Autodesk Fusion 360 part; units mm, degrees
sketch "Sketch1" plane through (0, 0, 0) normal (0, 0, 1) x (1, 0, 0)
  line L0 (0, 0) -> (51.8, 0)
  line L1 (51.8, 0) -> (51.8, 24.3)
  line L2 (51.8, 24.3) -> (0, 24.3)
  line L3 (0, 24.3) -> (0, 0)
  circle A0 centre (14, 5.4) radius 1.6
  circle A1 centre (38.7, 17.8) radius 1.6
  circle A2 centre (38.7, 5.4) radius 1.6
  line L4 (38.7, 17.8) -> (38.7, 5.4) construction
  line L5 (38.7, 5.4) -> (14, 5.4) construction
  line L6 (25.9, 24.3) -> (25.9, 0) construction
  circle A3 centre (38.7, 17.8) radius 3
  circle A4 centre (38.7, 5.4) radius 3
  circle A5 centre (14, 5.4) radius 3
  line L7 (51.8, 0) -> (59, 4.65)
  line L8 (59, 4.65) -> (59, 19.65)
  line L9 (59, 19.65) -> (51.8, 24.3)
  line L10 (0, 0) -> (-7.2, 4.65)
  line L11 (-7.2, 4.65) -> (-7.2, 19.65)
  line L12 (-7.2, 19.65) -> (0, 24.3)
  circle A6 centre (54.8, 12.15) radius 1.6
  circle A7 centre (-3, 12.15) radius 1.6
  line L13 (0, 12.15) -> (51.8, 12.15) construction
  circle A8 centre (-3, 12.15) radius 3
  circle A9 centre (54.8, 12.15) radius 3
  line L14 (-7.2, 4.65) -> (-10.8, 6.975)
  line L15 (-10.8, 6.975) -> (-10.8, 17.325)
  line L16 (-10.8, 17.325) -> (-8, 19.1333)
  line L17 (-8, 19.1333) -> (-8, 17.1333)
  line L18 (-8, 17.1333) -> (-8.8, 17.1333)
  line L19 (-8.8, 17.1333) -> (-8.8, 8.0642)
  line L20 (-8.8, 8.0642) -> (-7.2, 7.0308)
  dimension "d1" = 3.2
  dimension "d2" = 24.7
  dimension "d3" = 12.4
  dimension "d4" = 51.8
  dimension "d5" = 24.3
  dimension "d6" = 11.9
  dimension "d7" = 5.4
  dimension "d8" = 6
  dimension "d13" = 3.2
  dimension "d14" = 1.2
  dimension "d15" = 1.2
  dimension "d16" = 15
  dimension "d35" = 2
  dimension "d36" = 2
  dimension "d37" = 1.6
  dimension "d38" = 0.8
  dimension "d39" = 2
extrude "Extrude1" add sketch "Sketch1" along normal blind 5.6 contours L0 L1 L2 L3 | L3 L10 L11 L12 | L1 L7 L8 L9 | L11 L14 L15 L16 L17 L18 L19 L20
extrude "Extrude2" add sketch "Sketch1" along normal blind 2.5 contours A3 | A4 | A5
extrude "Extrude3" add sketch "Sketch1" along normal blind 2.6 from surface at 3 contours A8 | A9
sketch "Sketch2" plane through (0, 0, 5.6) normal (0, 0, 1) x (-1, 0, 0)
  circle A0 centre (-14, -5.4) radius 3
  circle A1 centre (-38.7, -17.8) radius 3
  circle A2 centre (-38.7, -5.4) radius 3
  line L0 (0, 0) -> (-51.8, 0)
  line L1 (-51.8, -24.3) -> (0, -24.3)
  line L2 (0, -24.3) -> (7.2, -19.65)
  line L3 (7.2, -19.65) -> (7.2, -7.0308)
  line L4 (10.8, -6.975) -> (0, 0)
  line L5 (-59.2, -13.3404) -> (7.2, -13.3404) construction
  line L6 (-59.2, -17.3404) -> (7.2, -17.3404)
  line L7 (7.2, -9.3404) -> (-59.2, -9.3404)
  line L8 (-51.5, -9.3404) -> (-51.5, -17.3404)
  line L9 (-0.5, -9.3404) -> (-0.5, -17.3404)
  line L10 (7.2, -7.0308) -> (8.8, -8.0642)
  line L11 (8.8, -8.0642) -> (8.8, -17.1333)
  line L12 (8.8, -17.1333) -> (8, -17.1333)
  line L13 (8, -17.1333) -> (8, -19.1333)
  line L14 (8, -19.1333) -> (10.8, -17.325)
  line L15 (10.8, -17.325) -> (10.8, -6.975)
  line L16 (-51.8, 0) -> (-59, -4.65)
  line L17 (-59, -4.65) -> (-59, -19.65)
  line L18 (-59, -19.65) -> (-51.8, -24.3)
  circle A3 centre (-54.8, -12.15) radius 1.6
  circle A4 centre (3, -12.15) radius 1.6
  dimension "d20" = 8
extrude "Extrude4" add sketch "Sketch2" along normal blind 1.2 contours A1 L6 L7 L8 L9
chamfer "Chamfer1" distance 1.2 angle 45 5 edges at (18.1177, 17.3404, 6.8) (26, 9.3404, 6.8) (46.5823, 17.3404, 6.8) (51.5, 13.3404, 6.8) (0.5, 13.3404, 6.8)
fillet "Fillet1" radius 1 2 edges at (-8.8, 12.5988, 0) (-7.2, 13.3404, 5.6)
equation "d7 = 4.2 mm + 1.2 mm"
equation "d15 = d14"
equation "d36 = d35"
equation "d39 = d35"
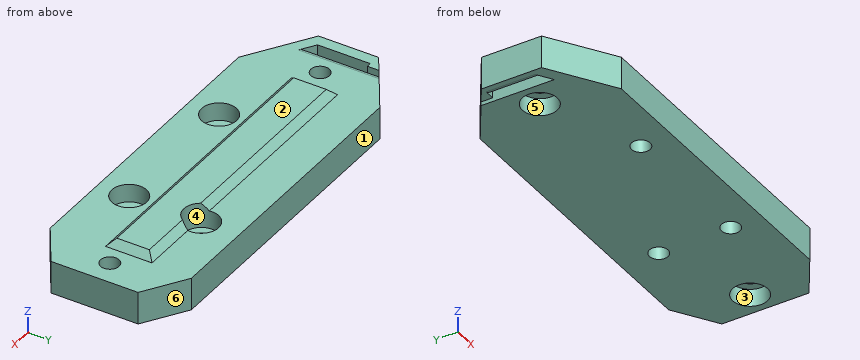
Geometry check sheet. Reference: the model listing, model coordinates, mm. Face numbers are marked on the shaded views. A direction names the side the tool comes from. Give positions to 0.01 mm unless a question says otherwise; leave off trailing zeros. Order: outer loops, then holes, each group sorted by start corner. A loop starts at its lowest first (then second) coordinate and runs counter-clockwise, first axis right, second up.
1. Section check A-A, the plane x = 38.7. Give the number of separate pieces and of enclosed holes in the cut face, and give its area (3 significant figures).
2. Access from +Z, -Z, +X, -X, +Y, -Y to the whole of each face (thin tool, end or side, straight path). Record for the marked faces 4, 5 and 6.
3. Thickness scan on L1, parallel to Y at x = 38.5, z = 3.25; L2, parallel to X at y = 6.5, z = 2.25; L3, parallel to X at y = 6.75, z = 1.75. Record the ranges inside material, lowest first.
4. Gauge pin test, flat ends, axial feed: pin 1 Ø4 at (x, y) = (-3, 12.15) entering from -Z; pin 2 Ø6.5 at (x, y) = (14.5, 4) entering from +Z; pin 3 Ø1.9 at (x, y) = (38.7, 5.4) entering from +Z; pin 4 Ø3.5 at (x, y) = (38.7, 17.8) entering from +Z. Record the tip position at first contact, or that the pin passes through.
5. Section check C-C, the plane z = 3.75. Enter the section's corners in (x, y) (3 decimals), and give its area (3 significant figures).
6. Release check for a two-part mould opening along Y. For the marked faces 1, 2 and 3 record: pulls with the +Y half, pulls with the -Y half, needs draft (parallel to the pull), parting line crosses it, or undercut.
Values follow:
1. separate pieces: 3
1. enclosed holes: 0
1. area: 88.7 mm2
2. face 4: +Z
2. face 5: -Z
2. face 6: +Z, -Z, +X, +Y
3. L1: y = 0 to 2.41, 8.39 to 14.81, 20.79 to 24.3
3. L2: x = -10.06 to 12.84, 15.16 to 37.54, 39.86 to 59
3. L3: x = -10.45 to 13.14, 14.86 to 37.84, 39.56 to 59
4. pin 1: stops at z = 3
4. pin 2: stops at z = 5.6
4. pin 3: passes through
4. pin 4: stops at z = 2.5
5. outline: (-10.8, 6.975) - (0, 0) - (51.8, 0) - (59, 4.65) - (59, 19.65) - (51.8, 24.3) - (0, 24.3) - (-7.2, 19.65) - (-7.2, 7.031) - (-8.8, 8.064) - (-8.8, 17.133) - (-8, 17.133) - (-8, 19.133) - (-10.8, 17.325) - close; hole circle Ø3.2 at (-3, 12.15); hole circle Ø6 at (14, 5.4); hole circle Ø6 at (38.7, 5.4); hole circle Ø6 at (38.7, 17.8); hole circle Ø3.2 at (54.8, 12.15)
5. area: 1,470 mm2
6. face 1: pulls with the +Y half
6. face 2: needs draft
6. face 3: undercut
